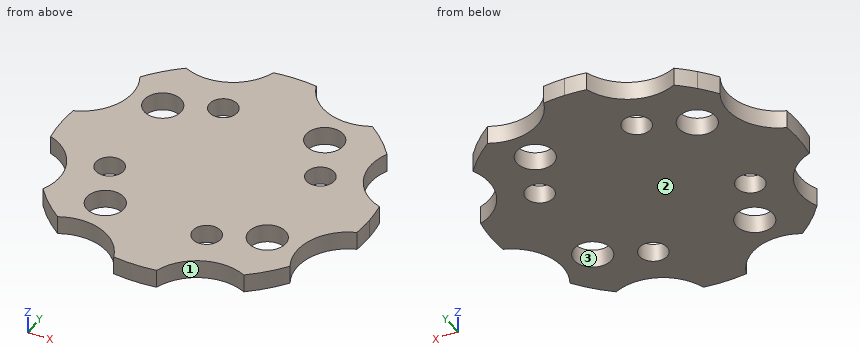
from build123d import *

# Parameters (mm, degrees)
BOSS_EXTRUDE1_DEPTH = 2
SKETCH2_R           = 1.5
SKETCH2_R_2         = 2
CUT_EXTRUDE1_DEPTH  = 24.420076857


with BuildPart() as part:
    # Sketch1 → Boss-Extrude1 (new body)
    with BuildSketch(Plane.XY):
        with BuildLine():
            ThreePointArc((2.29187449, 16.340052366), (1.148724502, 16.459964521), (0, 16.5))
            Line((0, 16.5), (0, 0))
            Line((0, 0), (-11.66726189, 11.66726189))
            ThreePointArc((-11.66726189, 11.66726189), (-12.451223415, 10.826681646), (-13.174761826, 9.933561839))
            ThreePointArc((-13.174761826, 9.933561839), (-13.026151447, 5.395608595), (-16.340052366, 2.29187449))
            ThreePointArc((-16.340052366, 2.29187449), (-16.5, 0), (-16.340052366, -2.29187449))
            ThreePointArc((-16.340052366, -2.29187449), (-13.026151447, -5.395608595), (-13.174761826, -9.933561839))
            ThreePointArc((-13.174761826, -9.933561839), (-11.66726189, -11.66726189), (-9.933561839, -13.174761826))
            ThreePointArc((-9.933561839, -13.174761826), (-5.395608595, -13.026151447), (-2.29187449, -16.340052366))
            ThreePointArc((-2.29187449, -16.340052366), (0, -16.5), (2.29187449, -16.340052366))
            ThreePointArc((2.29187449, -16.340052366), (5.395608595, -13.026151447), (9.933561839, -13.174761826))
            ThreePointArc((9.933561839, -13.174761826), (11.66726189, -11.66726189), (13.174761826, -9.933561839))
            ThreePointArc((13.174761826, -9.933561839), (13.026151447, -5.395608595), (16.340052366, -2.29187449))
            ThreePointArc((16.340052366, -2.29187449), (16.459964521, -1.148724502), (16.5, 0))
            ThreePointArc((16.5, 0), (16.459964521, 1.148724502), (16.340052366, 2.29187449))
            ThreePointArc((16.340052366, 2.29187449), (13.026151447, 5.395608595), (13.174761826, 9.933561839))
            ThreePointArc((13.174761826, 9.933561839), (11.66726189, 11.66726189), (9.933561839, 13.174761826))
            ThreePointArc((9.933561839, 13.174761826), (5.395608595, 13.026151447), (2.29187449, 16.340052366))
        make_face()
        with BuildLine():
            Line((0, 0), (0, 16.5))
            ThreePointArc((0, 16.5), (-1.148724502, 16.459964521), (-2.29187449, 16.340052366))
            ThreePointArc((-2.29187449, 16.340052366), (-5.395608595, 13.026151447), (-9.933561839, 13.174761826))
            ThreePointArc((-9.933561839, 13.174761826), (-10.826681646, 12.451223415), (-11.66726189, 11.66726189))
            Line((-11.66726189, 11.66726189), (0, 0))
        make_face()
    extrude(amount=BOSS_EXTRUDE1_DEPTH)

    # Sketch2 → Cut-Extrude1 (cut, through all)
    with BuildSketch(Plane.XY.offset(2)):
        with Locations((9.205631104, 3.905938552)):
            Circle(SKETCH2_R)
        with Locations((6.922242286, 9.183276198)):
            Circle(SKETCH2_R_2)
        with Locations((9.183276198, -6.922242286)):
            Circle(SKETCH2_R_2)
        with Locations((3.905938552, -9.205631104)):
            Circle(SKETCH2_R)
        with Locations((-6.922242286, -9.183276198)):
            Circle(SKETCH2_R_2)
        with Locations((-9.205631104, -3.905938552)):
            Circle(SKETCH2_R)
        with Locations((-9.183276198, 6.922242286)):
            Circle(SKETCH2_R_2)
        with Locations((-3.905938552, 9.205631104)):
            Circle(SKETCH2_R)
    extrude(amount=-CUT_EXTRUDE1_DEPTH, mode=Mode.SUBTRACT)


solid = part.part
Geometry: final body of the model. Coordinates: model frame, mm. Face numbers are marked on the shaded views. Coordinates: 2 decimals unless noted, no trailing zeros. Order: outer loops, then holes, each group sorted by start corner. A loop starts at its lowest first (then second) coordinate and runs counter-clockwise, first axis right, second up. Notation, with made-up numbers: (87.25, -21.5) - (119.25, -21.5) arc R18 ccw to (119.25, 11.5) - close; hole circle Ø4 at (78.25, 4.25). An arc over 180 degrees is marked (long way). Use one line per item in the form item = value.
1) Section D-D (x = 12). Return loops of the section in (y, z).
Solutions:
outline = (-11.32, 0) - (11.32, 0) - (11.32, 2) - (-11.32, 2) - close
2) Section C-C (z = 1.15). State how many separate pieces and enclosed holes the cut face has, then the cut area to 3 significant figures.
Solutions:
separate_pieces = 1
enclosed_holes = 8
area = 667 mm^2
3) Section A-A (x = -3.5). Return loops of the section in (y, z), then the cut area to 3 significant figures.
Solutions:
outline = (-14.33, 0) - (7.76, 0) - (7.76, 2) - (-14.33, 2) - close; (10.65, 0) - (14.33, 0) - (14.33, 2) - (10.65, 2) - close
area = 51.6 mm^2
4) Pin query (flat end, axial travel): pin 1 (6.5 mm diameter, centred on x = -9.18, y = 6.92, fed in from -Z); pin 2 (1.8 mm diameter, centred on x = -9.21, y = -3.91, fed in from +Z). Return the tip coordinate at first contact, or that it passes through.
Solutions:
pin_1 = 0
pin_2 = through
5) Mould query, pull axis Y, two halves, no side actions, for the marked faces 1, 2 and 3. Classes: +Y half, -Y half, draft (parallel to the pull), parting line (faces both ways), or undercut.
Solutions:
face_1 = -Y half
face_2 = draft
face_3 = undercut
6) Section B-B (y = 4.5). Return loops of the section in (x, z).
Solutions:
outline = (-13.5, 0) - (7.83, 0) - (7.83, 2) - (-13.5, 2) - close; (10.58, 0) - (13.5, 0) - (13.5, 2) - (10.58, 2) - close
7) Ray query, L1, parallel to Y at x = -10, z = 1.15; L2, parallel to Y at x = -9.5, z = 0.7; L3, parallel to X at y = -4.5, z = 0.5. Return the intervals inside material, ascending.
Solutions:
L1 = -13.12 to -5.18, -2.63 to 5.1, 8.75 to 13.12
L2 = -12.98 to -5.38, -2.44 to 4.95, 8.9 to 12.98
L3 = -13.5 to -10.58, -7.83 to 13.5
